Build history of the part. All positions in model axes, mm. Round coordinates to 2 decimals unless told otherwise and drop trailing zeros. Write each loop counter-clockwise with the first axis right and the second up, starting at its lowest first coordinate (ties: lowest second). Pieces come first, ordered by that corner, then holes. Notation, with made-up numbers: (-21, -7) - (8, -7) arc R12 ccw to (8, 12) - close; hole circle Ø4 at (49.5, 49.25). An arc over 180 degrees is marked (long way). Write each question's results on one line, items separated by ' | '.
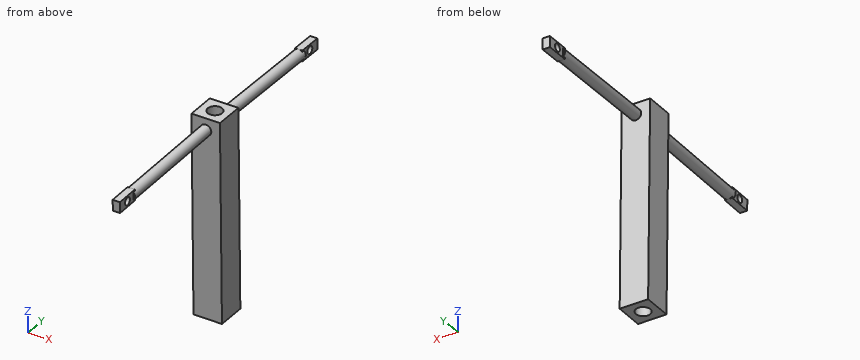
from build123d import *

# Parameters (mm, degrees)
SKETCH1_W           = 78.592769499
SKETCH1_H           = 78.592769498
SKETCH1_R           = 20
BOSS_EXTRUDE4_DEPTH = 550
SWEEP1_PROFILE_R    = 15
SKETCH15_R          = 10.5
BOSS_EXTRUDE5_DEPTH = 10


with BuildPart() as part:
    # Sketch1 → Boss-Extrude4 (new body)
    with BuildSketch(Plane(origin=(4e-09, 27232.877627093, 41716.336726155), x_dir=(1, 0, 0), z_dir=(0, -0.01550283, 0.999879824))):
        with Locations((-23373.04698752, 6409.461295652)):
            Rectangle(SKETCH1_W, SKETCH1_H)
        with Locations((-23373.046987519, 6409.461295652)):
            Circle(SKETCH1_R, mode=Mode.SUBTRACT)
    extrude(amount=-BOSS_EXTRUDE4_DEPTH)

    # Sweep1: sweep along a curve in space
    with BuildLine() as sweep1_path:
        Line((-23373.046987515, 34006.895340042, 41784.248904534), (-23373.046987515, 33681.357429633, 41784.248904534))
    # Sweep1 profile (on start of the path) → Sweep1 (sweep)
    with BuildSketch(Plane(origin=(-23373.046987515, 34006.895340042, 41784.248904534), x_dir=(0, 0, -1), z_dir=(0, -1, 0))):
        Circle(SWEEP1_PROFILE_R)
    sweep1 = sweep(path=sweep1_path.line)

    # Sketch15 → Boss-Extrude5 (add, symmetric)
    with BuildSketch(Plane(origin=(-23373.046987519, 0, 3e-09), x_dir=(0, 0, 1), z_dir=(-1, 0, 0))):
        Polygon((41769.248904556, 34063.932408428), (41799.248904531, 34063.932408428), (41799.248904531, 33999.858271629), (41769.248904531, 33999.858271629), align=None)
        with Locations((41784.248904537, 34031.895340042)):
            Circle(SKETCH15_R, mode=Mode.SUBTRACT)
    boss_extrude5 = extrude(amount=BOSS_EXTRUDE5_DEPTH, both=True)

    # Mirror1: Sweep1, Boss-Extrude5 across plane
    add(sweep1.mirror(Plane(origin=(0, 34281.667133734, 531.526740505), x_dir=(0, -0.01550283, 0.999879824), z_dir=(0, -0.999879824, -0.01550283))))
    add(boss_extrude5.mirror(Plane(origin=(0, 34281.667133734, 531.526740505), x_dir=(0, -0.01550283, 0.999879824), z_dir=(0, -0.999879824, -0.01550283))))


solid = part.part
(1) Drill centre lines: probe 1 along Y at (x, z) = (-23366.5, 41778.5); probe 2 along Y at (x, z) = (-23345, 41789); probe 3 along Y at (x, z) = (-23359.5, 41619). Where is each one in solid material? Low to high. Write a range as [from, to].
Worked answers:
probe 1: y = [33220.16, 33244.03], [33260.78, 33623.25], [33661.05, 34023.11], [34040.68, 34063.93] | probe 2: y = [33602.68, 33681.28] | probe 3: y = [33605.32, 33629.9], [33659.33, 33683.92]
(2) Flat gauge pins, fed straight in: pin 1 Ø9 at (y, z) = (34031, 41783) entering from -X; pin 2 Ø8 at (x, y) = (-23361.5, 33604) entering from +Z; pin 3 Ø3 at (x, y) = (-23361, 33723) entering from -Z; pin 4 Ø3 at (x, z) = (-23377, 41771) entering from -Y. Where does each tip first touch, or does it go through?
Worked answers:
pin 1: passes through | pin 2: stops at z = 41815.18 | pin 3: stops at z = 41773.58 | pin 4: stops at y = 33220.34
(3) Slice it at A-A, the plane x = -23403. Write the cut outline in (y, z).
Worked answers:
outline: (33602.28, 41815.09) - (33610.8, 41265.16) - (33689.39, 41266.38) - (33680.86, 41816.31) - close
